Could you check a few things on this drawing? It's one solid part, dimensions in mm from its lowest x, y, z. A direction names the side the tool comes from. Coordinates: 2 decimals unless noted, no trailing zeros. Order: outer loops, then holes, each group sorted by start corner. A loop starts at its lowest first (then second) coordinate and runs counter-clockwise, first axis right, second up. Notation, with made-up numbers: (-9, -9.75) -> (40, -9.75) arc R28 ccw to (40, 10.25) -> close; hole circle Ø9 at (-30.5, -35). An arc over 180 degrees is marked (long way). Use a Markdown table: item, result. Add a question column.
1. Suppose I cut it at D-D, the plane x = 5.25. List the corners of the cut face in (y, z) for me (3 decimals).
2. For pin 1 Ø4 at (x, y) = (17.35, 11.5) entering from +Z; pin 2 Ø2.5 at (y, z) = (4.5, 20) entering from -X; pin 3 Ø11 at (x, y) = (17, 18) entering from +Z; pin 4 Ø5 at (x, y) = (25.5, 5.5) entering from -Z, each with a flat end and sliding along its axis, tell me the tip position at first contact or that it passes through.
3. We'd pull the mould along X, two halves only. Please class the marked faces 5, 6 and 7: pulls with the +X half, pulls with the -X half, needs draft (parallel to the pull), parting line crosses it, or undercut.
4. Suppose I cut it at A-A, the plane z = 2.25. List the corners of the cut face in (x, y) for me.
5. For the marked faces 1, 2, 3 and 4, which set-ups out of +Z, -Z, +X, -X, +Y, -Y let a thin tool reach every point of the face, with its end or its side?
6. Suppose I cut it at C-C, the plane y = 5. List the corners of the cut face in (x, z) for me.
7. Suppose I cut it at B-B, the plane x = 10.35. List the corners of the cut face in (y, z) for me, then the cut area to 3 significant figures.
8. If I drill on line 1 along Y through (x, z) = (10.35, 2.5); line 2 along X through (y, z) = (18.5, 4); line 3 along X through (y, z) = (18.5, 0.7), over which ranges is the centre line in solid material (lowest first)? Write a range as from..to.
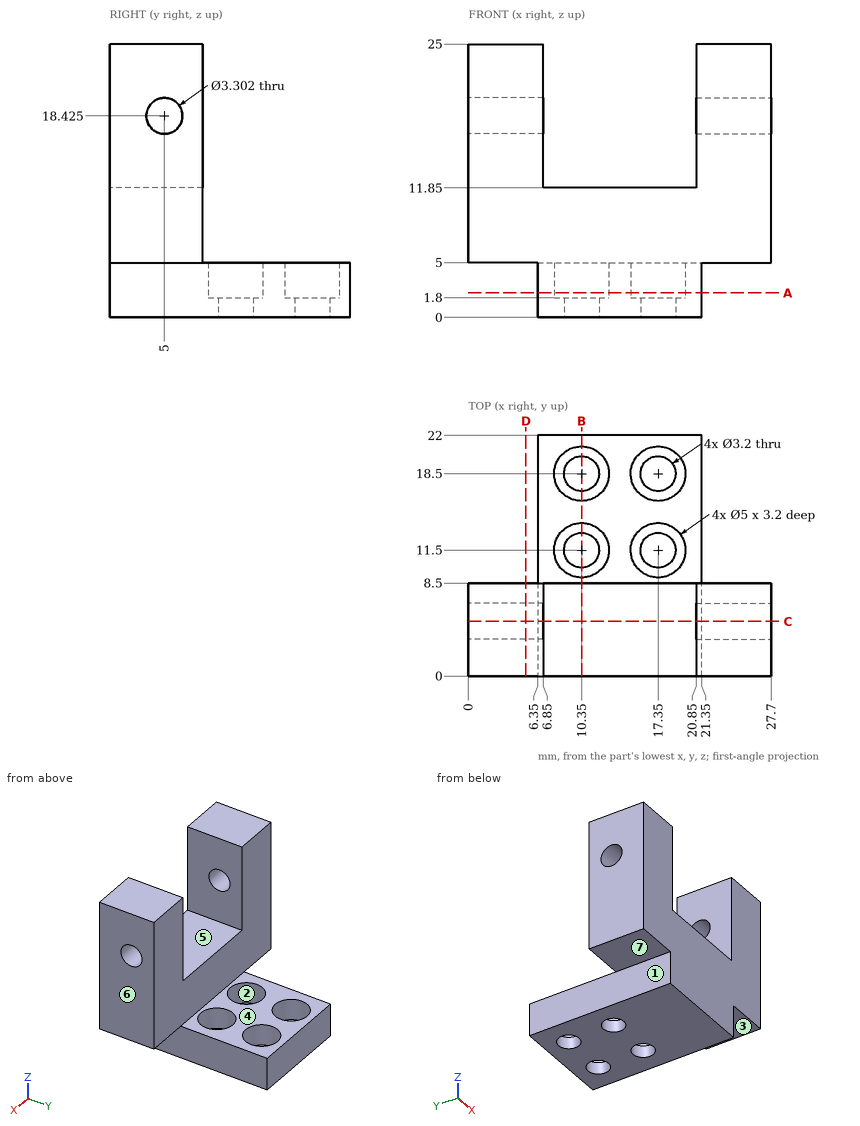
Worked out:
| question | item | result |
|---|---|---|
| 1 | outline | (0, 5) -> (8.5, 5) -> (8.5, 25) -> (0, 25) -> close; hole circle Ø3.302 at (5, 18.425) |
| 2 | pin 1 | stops at z = 1.8 |
| 2 | pin 2 | stops at x = 0 |
| 2 | pin 3 | stops at z = 5 |
| 2 | pin 4 | stops at z = 5 |
| 3 | face 5 | undercut |
| 3 | face 6 | pulls with the +X half |
| 3 | face 7 | needs draft |
| 4 | outline | (6.35, 0) -> (21.35, 0) -> (21.35, 22) -> (6.35, 22) -> close; hole circle Ø5 at (10.35, 11.5); hole circle Ø5 at (10.35, 18.5); hole circle Ø5 at (17.35, 11.5); hole circle Ø5 at (17.35, 18.5) |
| 5 | face 1 | -Z, -X, +Y, -Y |
| 5 | face 2 | +Z |
| 5 | face 3 | -Z, +X, +Y, -Y |
| 5 | face 4 | +Z, +X, -X, +Y |
| 6 | outline | (0, 5) -> (6.35, 5) -> (6.35, 0) -> (21.35, 0) -> (21.35, 5) -> (27.7, 5) -> (27.7, 16.77) -> (20.85, 16.77) -> (20.85, 11.85) -> (6.85, 11.85) -> (6.85, 16.77) -> (0, 16.77) -> close; (0, 20.08) -> (6.85, 20.08) -> (6.85, 25) -> (0, 25) -> close; (20.85, 20.08) -> (27.7, 20.08) -> (27.7, 25) -> (20.85, 25) -> close |
| 7 | outline | (0, 0) -> (9.9, 0) -> (9.9, 1.8) -> (9, 1.8) -> (9, 5) -> (8.5, 5) -> (8.5, 11.85) -> (0, 11.85) -> close; (13.1, 0) -> (16.9, 0) -> (16.9, 1.8) -> (16, 1.8) -> (16, 5) -> (14, 5) -> (14, 1.8) -> (13.1, 1.8) -> close; (20.1, 0) -> (22, 0) -> (22, 5) -> (21, 5) -> (21, 1.8) -> (20.1, 1.8) -> close |
| 7 | area | 125 mm² |
| 8 | line 1 | y = 0..9, 14..16, 21..22 |
| 8 | line 2 | x = 6.35..7.85, 12.85..14.85, 19.85..21.35 |
| 8 | line 3 | x = 6.35..8.75, 11.95..15.75, 18.95..21.35 |
